For this review, take the finished solid that the model builds, in its own axes (mm). Face numbers are marked on the shaded views. A direction names the side the tool comes from. Coordinates: 2 decimals unless noted, no trailing zeros. Loops run counter-clockwise (first coordinate to the right, second up) from the corner with the lowest first, then second, coordinate; pieces in that order, holes last. Notation, with made-up numbers: M 37.25,-23.75 L 72.25,-23.75 A18 cw 72.25,-4.75 Z; hole C -15.5,6 d7. An arc over 180 degrees is marked long. Put each result on its own line as item: value.
```python
from build123d import *


# Not quite as in the source:
# - a fillet or chamfer that OpenCascade refuses, or shapes differently, is made with other operations: its cross-section is extruded or revolved along the edge and cut away or added
# - ends of sketch curves that miss each other by under 0.0002 mm in the source are joined


with BuildPart() as f1:
    # F0 (on Front) → F1 (revolve)
    with BuildSketch(Plane.XZ):
        with BuildLine():
            Line((1.55, 10.5700949207), (1.55, 4.9207e-06))
            Line((1.55, 4.9207e-06), (22.5, 0))
            Line((22.5, 0), (22.5, 1.1))
            ThreePointArc((22.5, 1.1), (20.1, 3.5), (22.5, 5.9))
            Line((22.5, 5.9), (22.5, 7))
            Line((22.5, 7), (3.9362940006, 7))
            Line((3.9362940006, 7), (3.9362940006, 10.5700949207))
            Line((3.9362940006, 10.5700949207), (1.55, 10.5700949207))
        make_face()
    revolve(axis=Axis((0, 0, 5.2850474603), (0, 0, -1)))

    # F2: fillet of radius 5 on 1 edges, made by hand

    # F2_s1 → F2_t2 (revolve)
    with BuildSketch(Plane.XZ):
        with BuildLine():
            ThreePointArc((8.7274704182, 7), (5.739956853, 7.9906655542), (3.9362940006, 10.5700949207))
            Line((3.9362940006, 10.5700949207), (3.9362940006, 7))
            Line((3.9362940006, 7), (8.7274704182, 7))
        make_face()
    revolve(axis=Axis((0, 0, 7), (0, 0, -1)))


solid = f1.part
```
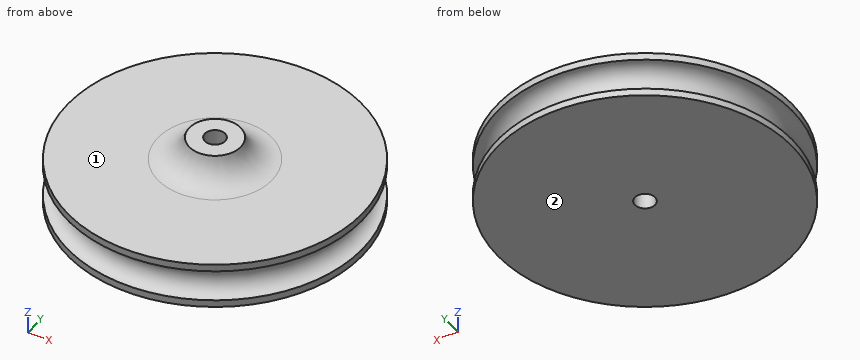
(1) Tool access review of the marked faces 1 and 2: name each direction out of +Z, -Z, +X, -X, +Y, -Y from which nothing blocks a thin tool from reaching the whole face with its end or side.
Determined:
face 1: +Z
face 2: -Z, +X, -X, +Y, -Y
(2) Add section A-A (y = 0). Write out the cut boundary in (x, z), plus the area to 3 significant figures.
Determined:
outline: M -22.5,0 L -1.55,0 L -1.55,10.57 L -3.94,10.57 A5 cw -8.73,7 L -22.5,7 L -22.5,5.9 A2.4 cw -22.5,1.1 Z; M 1.55,0 L 22.5,0 L 22.5,1.1 A2.4 cw 22.5,5.9 L 22.5,7 L 8.73,7 A5 cw 3.94,10.57 L 1.55,10.57 Z
area: 301 mm^2
(3) Wall thickness on line 1 along Z through (x, y) = (1, 9); line 2 along Z through (x, y) = (-16, -13); line 3 along Y through (x, z) = (0, 5.25): over which ranges is each line inside the solid? List them lowest first. Write a range as [from, to].
Determined:
line 1: z = [0, 7]
line 2: z = [0, 2.01], [4.99, 7]
line 3: y = [-20.86, -1.55], [1.55, 20.86]
(4) Add section C-C (z = 4.75). Write out the cut boundary in (x, y), plus the area to 3 significant figures.
Determined:
outline: C 0,0 d40.9; hole C 0,0 d3.1
area: 1,310 mm^2
(5) For pin 1 (2 mm diameter, centred on x = 16.5, z = 4.5, fed in from +Y); pin 2 (4 mm diameter, centred on x = -16, y = -17.5, fed in from -Z); pin 3 (1.5 mm diameter, centred on y = -13, z = 5.5, fed in from +X); pin 4 (1.5 mm diameter, centred on y = 15, z = 4, fed in from +X), all flat-tipped, find the tip position at first contact; note any pin that passes through.
Determined:
pin 1: stops at y = 13.59
pin 2: stops at z = 0
pin 3: stops at x = 18.8
pin 4: stops at x = 14.31
